```python
from build123d import *

# Parameters (mm, degrees)
F0_R     = 11.2
F0_R_2   = 3
F0_R_3   = 2.5
F0_R_4   = 2
F1_DEPTH = 7


# Not quite as in the source:
# - a feature names something its author has since deleted; it is built from what else it names


with BuildPart() as f1:
    # F0 (on Top) → F1 (new body)
    with BuildSketch(Plane.XY):
        with BuildLine():
            ThreePointArc((-6.1736201838, 37.9133765769), (-7.7319005407, 36.9445453014), (-9.1407759551, 35.7689851037))
            ThreePointArc((-9.1407759551, 35.7689851037), (-7.6864399565, 36.8816423115), (-6.1736201838, 37.9133765769))
        make_face()
        with BuildLine():
            ThreePointArc((-26.4064617899, -25.8006367392), (-28.0972191968, -25.0974734227), (-29.7471371669, -24.3032002009))
            ThreePointArc((-29.7471371669, -24.3032002009), (-28.1289644919, -25.1682949385), (-26.4064617899, -25.8006367392))
        make_face()
        with BuildLine():
            ThreePointArc((35.929749598, -13.123027049), (35.8337727119, -11.5341349098), (35.5472377449, -9.9683483645))
            ThreePointArc((35.5472377449, -9.9683483645), (35.7836591533, -11.7841688888), (35.9207573507, -13.610176376))
            ThreePointArc((35.9207573507, -13.610176376), (35.9275013447, -13.3666432057), (35.929749598, -13.123027049))
        make_face()
        with BuildLine():
            ThreePointArc((-6.1736201838, 37.9133765769), (-7.6864399565, 36.8816423115), (-9.1407759551, 35.7689851037))
            ThreePointArc((-9.1407759551, 35.7689851037), (-13.1996365954, 26.3440017791), (-9.2810910796, 16.8598222464))
            ThreePointArc((-9.2810910796, 16.8598222464), (-5.669005002, 14.3253837189), (-1.4234328474, 13.123027049))
            ThreePointArc((-1.4234328474, 13.123027049), (0, 13.2), (1.4234328474, 13.123027049))
            ThreePointArc((1.4234328474, 13.123027049), (9.824187335, 17.4298563231), (13.2, 26.246054098))
            ThreePointArc((13.2, 26.246054098), (6.8098536539, 37.5538343052), (-6.1736201838, 37.9133765769))
        make_face()
        with Locations((0, 26.246054098)):
            Circle(F0_R, mode=Mode.SUBTRACT)
        with BuildLine():
            ThreePointArc((-10.6531583753, -7.7942425309), (-11.43153533, -6.6), (-12.0765912227, -5.3287845181))
            ThreePointArc((-12.0765912227, -5.3287845181), (-32.389553942, -4.1270179319), (-29.7471371669, -24.3032002009))
            ThreePointArc((-29.7471371669, -24.3032002009), (-28.0972191968, -25.0974734227), (-26.4064617899, -25.8006367392))
            ThreePointArc((-26.4064617899, -25.8006367392), (-16.2147564803, -24.6032215019), (-9.9604888289, -16.467571773))
            ThreePointArc((-9.9604888289, -16.467571773), (-9.6378772691, -14.8091109508), (-9.529749598, -13.123027049))
            ThreePointArc((-9.529749598, -13.123027049), (-9.8136549069, -10.4000694786), (-10.6531583753, -7.7942425309))
        make_face()
        with Locations((-22.729749598, -13.123027049)):
            Circle(F0_R, mode=Mode.SUBTRACT)
        with BuildLine():
            ThreePointArc((35.5472377449, -9.9683483645), (29.4143930758, -1.7407802772), (19.2415799085, -0.3922504734))
            ThreePointArc((19.2415799085, -0.3922504734), (15.2406487206, -2.2531895135), (12.0765912227, -5.3287845181))
            ThreePointArc((12.0765912227, -5.3287845181), (11.43153533, -6.6), (10.6531583753, -7.7942425309))
            ThreePointArc((10.6531583753, -7.7942425309), (19.7688793419, -25.9866675651), (35.9207573507, -13.610176376))
            ThreePointArc((35.9207573507, -13.610176376), (35.7836591533, -11.7841688888), (35.5472377449, -9.9683483645))
        make_face()
        with Locations((22.729749598, -13.123027049)):
            Circle(F0_R, mode=Mode.SUBTRACT)
        with BuildLine():
            ThreePointArc((-1.4234328474, 13.123027049), (-5.669005002, 14.3253837189), (-9.2810910796, 16.8598222464))
            ThreePointArc((-9.2810910796, 16.8598222464), (-26.9770057804, 0.3443606169), (-46.801379663, 14.2332075847))
            ThreePointArc((-46.801379663, 14.2332075847), (-45.0709674202, -8.0428719823), (-29.7471371669, -24.3032002009))
            ThreePointArc((-29.7471371669, -24.3032002009), (-32.389553942, -4.1270179319), (-12.0765912227, -5.3287845181))
            ThreePointArc((-12.0765912227, -5.3287845181), (-11.43153533, 6.6), (-1.4234328474, 13.123027049))
        make_face()
        with Locations((-39.597851646, -5.3848865237)):
            Circle(F0_R_2, mode=Mode.SUBTRACT)
        with Locations((-42.7842679926, 0.1341484827)):
            Circle(F0_R_3, mode=Mode.SUBTRACT)
        with Locations((-45.0379561931, 5.4032604173)):
            Circle(F0_R_4, mode=Mode.SUBTRACT)
        with BuildLine():
            ThreePointArc((35.7270091772, 33.4145799279), (15.570152254, 43.0540387502), (-6.1736201838, 37.9133765769))
            ThreePointArc((-6.1736201838, 37.9133765769), (6.8098536539, 37.5538343052), (13.2, 26.246054098))
            ThreePointArc((13.2, 26.246054098), (9.824187335, 17.4298563231), (1.4234328474, 13.123027049))
            ThreePointArc((1.4234328474, 13.123027049), (9.824187335, 8.816197775), (13.2, 0))
            ThreePointArc((13.2, 0), (12.9160946911, -2.7229575704), (12.0765912227, -5.3287845181))
            ThreePointArc((12.0765912227, -5.3287845181), (15.2406487206, -2.2531895135), (19.2415799085, -0.3922504734))
            ThreePointArc((19.2415799085, -0.3922504734), (13.7867279325, 23.1905920154), (35.7270091772, 33.4145799279))
        make_face()
        with Locations((15.135477297, 36.9851887226)):
            Circle(F0_R_2, mode=Mode.SUBTRACT)
        with Locations((21.5083099902, 36.9851887226)):
            Circle(F0_R_3, mode=Mode.SUBTRACT)
        with Locations((27.1983388811, 36.3023839891)):
            Circle(F0_R_4, mode=Mode.SUBTRACT)
        with BuildLine():
            ThreePointArc((10.6531583753, -7.7942425309), (0, -13.2), (-10.6531583753, -7.7942425309))
            ThreePointArc((-10.6531583753, -7.7942425309), (-9.8136549069, -10.4000694786), (-9.529749598, -13.123027049))
            ThreePointArc((-9.529749598, -13.123027049), (-9.6378772691, -14.8091109508), (-9.9604888289, -16.467571773))
            ThreePointArc((-9.9604888289, -16.467571773), (13.1902778479, -23.5349526323), (11.0743704858, -47.6477875127))
            ThreePointArc((11.0743704858, -47.6477875127), (29.5008151662, -35.0111667679), (35.9207573507, -13.610176376))
            ThreePointArc((35.9207573507, -13.610176376), (19.7688793419, -25.9866675651), (10.6531583753, -7.7942425309))
        make_face()
        with Locations((17.8396173119, -41.7056444063)):
            Circle(F0_R_4, mode=Mode.SUBTRACT)
        with Locations((21.2759580025, -37.1193372053)):
            Circle(F0_R_3, mode=Mode.SUBTRACT)
        with Locations((24.462374349, -31.6003021989)):
            Circle(F0_R_2, mode=Mode.SUBTRACT)
    extrude(amount=F1_DEPTH)


solid = f1.part
```
Verification items for the finished model (mm, model axes). A direction names the side the tool comes from. Give positions to 0.01 mm unless a question says otherwise; leave off trailing zeros. Loops run counter-clockwise (first coordinate to the right, second up) from the corner with the lowest first, then second, coordinate; pieces in that order, holes last.
1. Set-up check for faces 5 (the cylindrical face through (-26.612, 0.373, 3.451)), 6 (the flat face through (-6, -12, 0)): record each of +Z, -Z, +X, -X, +Y, -Y from which the full face is reachable in a straight line by a thin tool's end or side.
2. Section check C-C, the plane z = 3. Count the separate pieces of the cut face and the enclosed holes in it, then the cut area to 3 significant figures.
3. Section check D-D, the plane y = 32. Enter the section's corners in (x, z), then the cut area to 3 significant figures.
4. Section check A-A, the plane y = -33.5. Enter the section's corners in (x, z).
5. Section check B-B, the plane x = 0. Enter the section's corners in (y, z), then the cut area to 3 significant figures.
6. Mould release check, pull along Y, two halves, no side actions. Record for faces 1 (the flat face through (-6, -12, 7)), 2 (the cylindrical face through (17.91, 35.84, 3.45)), 3 (the cylindrical face through (15.89, 43.02, 3.45)), 4 (the cylindrical face through (12.98, -23.23, 3.45)): released by +Y, released by -Y, zero draft, split by the parting line, or undercut.
7. Thickness scan on line 1 (Y direction, x = -8, z = 6.25); line 2 (Y direction, x = -7, z = 5); line 3 (X direction, y = -10, z = 2.25). Record the ranges inside material, lowest first.
8. Go/stop test with flat-tipped pins: pin 1 Ø1.5 at (y, z) = (-20, 3) entering from +X; pin 2 Ø13.5 at (x, y) = (-22.73, -13.12) entering from +Z; pin 3 Ø3 at (x, z) = (-29, 1.5) entering from -Y; pin 4 Ø4 at (x, z) = (-8.5, 2) entering from -Y. Record where each tip stops, or that it passes through.
Geometry says:
1. face 5: +Z, -Z
1. face 6: -Z, +X, -X, +Y, -Y
2. separate pieces: 1
2. enclosed holes: 13
2. area: 1,380 mm2
3. outline: (-11.88, 0) - (-9.61, 0) - (-9.61, 7) - (-11.88, 7) - close; (9.61, 0) - (22.55, 0) - (22.55, 7) - (9.61, 7) - close
3. area: 106 mm2
4. outline: (16.46, 0) - (22.14, 0) - (22.14, 7) - (16.46, 7) - close; (26.78, 0) - (30.54, 0) - (30.54, 7) - (26.78, 7) - close
5. outline: (-15.26, 0) - (-13.2, 0) - (-13.2, 7) - (-15.26, 7) - close; (13.2, 0) - (15.05, 0) - (15.05, 7) - (13.2, 7) - close; (37.45, 0) - (41.03, 0) - (41.03, 7) - (37.45, 7) - close
5. area: 52.5 mm2
6. face 1: zero draft
6. face 2: undercut
6. face 3: released by +Y
6. face 4: undercut
7. line 1: y = -15.79 to -10.5, 10.5 to 18.41, 34.08 to 36.75
7. line 2: y = -15.54 to -11.19, 11.19 to 17.5, 34.99 to 37.44
7. line 3: x = -44.13 to -33.49, -11.97 to -8.62, 8.62 to 11.97, 33.49 to 35.55
8. pin 1: stops at x = 35.72
8. pin 2: passes through
8. pin 3: stops at y = -25.43
8. pin 4: stops at y = -18.09
